from build123d import *

# Parameters (mm, degrees)
SKETCH2_W           = 47.5
SKETCH2_H           = 31.66666
BOSS_EXTRUDE1_DEPTH = 43.5
DRAFT2_ANGLE        = -5
DRAFT3_ANGLE        = -5
DRAFT4_ANGLE        = -3
DRAFT5_ANGLE        = -3
FILLET1_R           = 6
FILLET2_R           = 2
SKETCH3_W           = 65.927175626
SKETCH3_H           = 41.406577606
CUT_EXTRUDE1_DEPTH  = 5.5


with BuildPart() as part:
    # Sketch2 → Boss-Extrude1 (new body)
    with BuildSketch(Plane(origin=(0, 0, 0), x_dir=(1, 0, 0), z_dir=(0, 1, 0))):
        Rectangle(SKETCH2_W, SKETCH2_H)
    extrude(amount=BOSS_EXTRUDE1_DEPTH)

    # Draft2
    draft2_faces = [part.faces().sort_by_distance(p)[0] for p in [
        (0, 21.75, 15.83333),
    ]]
    draft(draft2_faces, Plane.ZX.offset(43.5), DRAFT2_ANGLE)

    # Draft3
    draft3_faces = [part.faces().sort_by_distance(p)[0] for p in [
        (0, 21.75, -15.83333),
    ]]
    draft(draft3_faces, Plane.ZX.offset(43.5), DRAFT3_ANGLE)

    # Draft4
    draft4_faces = [part.faces().sort_by_distance(p)[0] for p in [
        (-23.75, 22.740338939, 0),
    ]]
    draft(draft4_faces, Plane.ZX.offset(43.5), DRAFT4_ANGLE)

    # Draft5
    draft5_faces = [part.faces().sort_by_distance(p)[0] for p in [
        (23.75, 22.740338939, 0),
    ]]
    draft(draft5_faces, Plane.ZX.offset(43.5), DRAFT5_ANGLE)

    # Fillet1
    fillet1_edges = [part.edges().sort_by_distance(p)[0] for p in [
        (21.470261601, 0, 0),
        (-21.470261601, 0, 0),
    ]]
    fillet(fillet1_edges, radius=FILLET1_R)

    # Fillet2
    fillet2_edges = [part.edges().sort_by_distance(p)[0] for p in [
        (23.75, 43.5, 0),
        (0, 43.5, -15.83333),
        (0, 0, 12.027573137),
        (19.910526358, 1.651481544, 12.17205905),
        (-19.910526358, 1.651481544, 12.17205905),
        (0, 0, -12.027573137),
        (19.910526358, 1.651481544, -12.17205905),
        (-19.910526358, 1.651481544, -12.17205905),
        (-23.75, 43.5, 0),
        (0, 43.5, 15.83333),
        (-22.759125705, 24.592992131, -14.17918115),
        (22.759125705, 24.592992131, -14.17918115),
        (22.759125705, 24.592992131, 14.17918115),
        (-22.759125705, 24.592992131, 14.17918115),
    ]]
    fillet(fillet2_edges, radius=FILLET2_R)

    # Sketch3 → Cut-Extrude1 (cut)
    with BuildSketch(Plane(origin=(0, 43.5, 0), x_dir=(1, 0, 0), z_dir=(0, 1, 0))):
        Rectangle(SKETCH3_W, SKETCH3_H)
    extrude(amount=-CUT_EXTRUDE1_DEPTH, mode=Mode.SUBTRACT)


solid = part.part
Geometry check sheet. Reference: the model listing, model coordinates, mm. Coordinates: 2 decimals unless noted, no trailing zeros. Order: outer loops, then holes, each group sorted by start corner. A loop starts at its lowest first (then second) coordinate and runs counter-clockwise, first axis right, second up. Notation, with made-up numbers: M 1,57 L 40,57 A31 ccw 40,90 Z; hole C 49,66 d9. An arc over 180 degrees is marked long. Use CSV: the item, a comma, the result in double quotes.
Item 1: Gauge pin test, flat ends, axial feed: pin 1 Ø1.5 at (x, y) = (-3.5, 20) entering from +Z; pin 2 Ø1.5 at (x, y) = (-18.5, 23) entering from +Z; pin 3 Ø8 at (x, y) = (11, 15) entering from +Z. Record the tip position at first contact, or that the pin passes through.
Returned:
pin 1,"stops at z = 13.84"
pin 2,"stops at z = 14.11"
pin 3,"stops at z = 13.69"
Item 2: Cross-section at A-A on z = -3.5. Record the cut outline in (x, y).
Returned:
outline,"M -23.46,38 L -21.77,5.69 A6 ccw -15.78,0 L 15.78,0 A6 ccw 21.77,5.69 L 23.46,38 Z"
Item 3: Cross-section at B-B on x = -9. Record the cut outline in (y, z).
Returned:
outline,"M 0,-10.19 A2 ccw 1.83,-12.19 L 38,-15.35 L 38,15.35 L 1.83,12.19 A2 ccw 0,10.19 Z"
Item 4: Thickness scan on line 1 along X through (y, z) = (5.5, -4.5); line 2 along X through (y, z) = (22, 4.5); line 3 along Y through (x, z) = (-18.5, 4.5). Record the ranges inside material, lowest first.
Returned:
line 1,"x = -21.76 to 21.76"
line 2,"x = -22.62 to 22.62"
line 3,"y = 0.65 to 38"
